Read the model definition and answer for the solid it produces. Units are mm, in the model's axes. A direction names the side the tool comes from. Coordinates: 2 decimals unless noted, no trailing zeros. Order: outer loops, then holes, each group sorted by start corner. A loop starts at its lowest first (then second) coordinate and runs counter-clockwise, first axis right, second up. Notation, with made-up numbers: M 39,74 L 80,74 A15 ccw 80,99 Z; hole C -28,-24.5 d10. An arc over 180 degrees is marked long. One line per question, with ' | ' between items. Start each with the question number.
1) Given P1, Ø3, axis at x = -7, z = -5, coming from the +Y side; P2, Ø2.5, axis at y = -2.5, z = 12, coming from the -X side; P3, Ø7, axis at y = 2.5, z = 10.5, coming from the +X side; P4, Ø1.5, axis at x = -3.5, z = 3.5, coming from the -Y side, each flat-ended and moving along its own axis, determine where each tip first touches the part or whether it passes through.
2) Find section D-D, the plane y = -13.75. Write down the section's boundary in (x, z), plus the area to 3 significant figures.
3) Consider probe 1 along Z at (x, y) = (-2.5, -12.5); probe 2 along Z at (x, y) = (-2, -10.5); probe 3 along X at (y, z) = (-6, 13.5). Determine where each line is inside the solid, lowest interval first.
4) Find section C-C, the plane x = -4. Write down the section's boundary in (y, z).
5) A tool of negligible diameter and unlimited length cuts with its end or side. For faces 1 (the face through (-3.3, 0, 10)), 2 (the face through (-10.116, 0.147, -4.181)), 3 (the face through (-12.66, -7.66, -7.47)), 4 (the face through (-14.8, 1.6, -5.7)), from which of +Z, -Z, +X, -X, +Y, -Y can it reach the whole face along a straight path? Write none if from no direction.
6) The mould has two halves that part along Z. Classify faces 5 (the face through (-5, -7, 15)), 6 (the face through (-4.21, -10.16, 11.3)), 7 (the face through (-2, -11, 6)), 8 (the face through (-13.02, -7.64, -9.05)): +Z half, -Z half, draft (parallel to the pull), parting line (faces both ways), or undercut.
7) Find section A-A, the plane y = 2. Write down the section's boundary in (x, z), plus the area to 3 significant figures.
8) Find section B-B, the plane z = 9.25. Write down the section's boundary in (x, y).
Solid Edge part; units mm, degrees
sketch "Sketch1" plane through (0, 0, 0) normal (0, -1, 0) x (1, 0, 0)
  line L0 (-8.3, 6) -> (-8.3, 15)
  line L1 (-8.3, 15) -> (-3.3, 15)
  line L2 (-3.3, 6) -> (-3.3, 15)
  line L3 (-3.3, 6) -> (-6.7175, -1.3288)
  line L4 (-6.7175, -1.3288) -> (-13.6119, -7.1139)
  line L5 (-16.8258, -3.2836) -> (-13.6119, -7.1139)
  line L6 (-9.9314, 2.5014) -> (-16.8258, -3.2836)
  line L7 (-8.3, 6) -> (-9.9314, 2.5014)
extrude "ExtrudedProtrusion_1" add sketch "Sketch1" along normal mid plane 16
sketch "Sketch2" plane through (0, -8, 0) normal (0, -1, 0) x (1, 0, 0)
  line L0 (-8.3, 15) -> (-3.3, 15)
  line L1 (-3.3, 6) -> (-3.3, 15)
  line L2 (-3.3, 6) -> (-11.969, -12.5907)
  line L3 (-16, -12.5907) -> (-11.969, -12.5907)
  line L4 (-16, -2.5907) -> (-16, -12.5907)
  line L5 (-16, -2.5907) -> (-9.9314, 2.5014)
  line L6 (-9.9314, 2.5014) -> (-8.3, 6)
  line L7 (-8.3, 6) -> (-8.3, 15)
extrude "Protrusion1" add sketch "Sketch2" along normal blind 9
sketch "Sketch3" plane through (-16, -11.5, 1.2046) normal (-1, 0, 0) x (0, -1, 0)
  circle A0 centre (-1.5, -9.4744) radius 2.2
extrude "Cutout1" cut sketch "Sketch3" against normal through all
sketch "Sketch4" plane through (-11.3587, -8, -6.9597) normal (0, 1, 0) x (0, 0, 1)
  line L0 (-5.631, -0.6103) -> (-5.631, -4.6413)
  line L1 (-5.631, -4.6413) -> (2.6919, -4.6413)
  line L2 (-0.1541, -2.2532) -> (2.6919, -4.6413)
  line L3 (5.631, 4.6412) -> (-0.1541, -2.2532)
  line L4 (5.631, 4.6412) -> (-5.631, -0.6103)
extrude "ExtrudedProtrusion_5" add sketch "Sketch4" along normal blind 3
sketch "Sketch5" plane through (-9.65, -17, 1.2046) normal (0, -1, 0) x (1, 0, 0)
  line L0 (-6.35, -13.7954) -> (-6.35, 13.7954)
extrude "Cutout2" cut sketch "Sketch5" against normal through all material side at (-16.05, -17, 1.2046)
sketch "Sketch6" plane through (-12.9657, -4.5, -0.0447) normal (-0.6427876, 0, 0.7660444) x (0.7660444, 0, 0.6427876)
  circle A0 centre (-0.539, 7) radius 2.2
extrude "Cutout3" cut sketch "Sketch6" against normal through all
sketch "Sketch7" plane through (-12.9657, -4.5, -0.0447) normal (-0.6427876, 0, 0.7660444) x (0.7660444, 0, 0.6427876)
  line L0 (-0.539, 7) -> (1.0435, 8.5282)
  line L1 (1.0435, 8.5282) -> (-0.539, 10.167)
  line L2 (-0.539, 10.167) -> (-2.1216, 8.5282)
  line L3 (-2.1216, 8.5282) -> (-0.539, 7)
extrude "Cutout4" cut sketch "Sketch7" against normal through all
sketch "Sketch8" plane through (-16, -4.5, -7.5907) normal (-1, 0, 0) x (0, 0, 1)
  line L0 (-0.6791, -5.5) -> (0.9035, -3.9718)
  line L1 (0.9035, -3.9718) -> (-0.6791, -2.333)
  line L2 (-0.6791, -2.333) -> (-2.2616, -3.9718)
  line L3 (-2.2616, -3.9718) -> (-0.6791, -5.5)
extrude "Cutout5" cut sketch "Sketch8" against normal through all
sketch "Sketch9" plane through (-3.3, -4.5, 10.5) normal (1, 0, 0) x (0, 0, -1)
  line L0 (4.5, -12.5) -> (-4.5, -12.5)
  line L1 (-4.5, -12.5) -> (-4.5, -0.5)
  line L2 (-4.5, -0.5) -> (4.5, -0.5)
  line L3 (4.5, -12.5) -> (4.5, -0.5)
  dimension "D1" = 4.5
extrude "ExtrudedProtrusion_4" add sketch "Sketch9" along normal blind 3.3
sketch "Sketch10" plane through (-8.3, -4.5, 10.5) normal (-1, 0, 0) x (0, 0, 1)
  circle A0 centre (0, 7) radius 2.2
  circle A1 centre (0, -8) radius 2.2
extrude "Cutout6" cut sketch "Sketch10" against normal through all
sketch "Sketch11" plane through (-8.3, -4.5, 10.5) normal (-1, 0, 0) x (0, 0, 1)
  line L0 (0, 7) -> (1.5825, 8.5282)
  line L1 (1.5825, 8.5282) -> (0, 10.167)
  line L2 (0, 10.167) -> (-1.5825, 8.5282)
  line L3 (-1.5825, 8.5282) -> (0, 7)
  line L4 (0, -8) -> (1.5825, -6.4718)
  line L5 (1.5825, -6.4718) -> (0, -4.833)
  line L6 (0, -4.833) -> (-1.5825, -6.4718)
  line L7 (-1.5825, -6.4718) -> (0, -8)
extrude "Cutout7" cut sketch "Sketch11" against normal through all
Report:
1) P1: stops at y = -5 | P2: stops at x = -8.3 | P3: stops at x = -3.3 | P4: passes through
2) outline: M -16,-12.59 L -11.97,-12.59 L -3.3,6 L 0,6 L 0,8.69 L -8.3,8.69 L -8.3,6 L -9.93,2.5 L -16,-2.59 Z; M -8.3,12.31 L 0,12.31 L 0,15 L -8.3,15 Z | area: 161 mm^2
3) probe 1: z = 6 to 8.3, 12.7 to 15 | probe 2: z = 6 to 9.37, 11.63 to 15 | probe 3: x = -8.3 to 0
4) outline: M -17,4.5 L 8,4.5 L 8,15 L -17,15 Z; hole M -10.97,8.92 L -9.33,10.5 L -10.97,12.08 A2.2 ccw long Z; hole M 4.03,8.92 L 5.67,10.5 L 4.03,12.08 A2.2 ccw long Z
5) face 1: +Z, -Z, +X, +Y | face 2: -Z, +X, +Y | face 3: +X, -X | face 4: -Z, -X, +Y
6) face 5: +Z half | face 6: undercut | face 7: -Z half | face 8: undercut
7) outline: M -16,-4.27 L -13.61,-7.11 L -11.81,-5.6 L -15.02,-1.77 L -16,-2.59 Z; M -11.74,0.99 L -8.52,-2.84 L -6.72,-1.33 L -3.3,6 L -3.3,8.36 L -8.3,8.36 L -8.3,6 L -9.93,2.5 Z; M -8.3,12.64 L -3.3,12.64 L -3.3,15 L -8.3,15 Z | area: 73.5 mm^2
8) outline: M -8.3,-17 L 0,-17 L 0,-14.31 L -8.3,-14.31 Z; M -8.3,-10.63 L 0,-10.63 L 0,-5 L -3.3,-5 L -3.3,0.69 L -8.3,0.69 Z; M -8.3,4.37 L -3.3,4.37 L -3.3,8 L -8.3,8 Z
